For this review, take the finished solid that the model builds, in its own axes (mm). A direction names the side the tool comes from. Give positions to 0.01 mm unless a question says otherwise; leave off trailing zeros. Write each loop counter-clockwise with the first axis right and the second up, starting at its lowest first coordinate (ties: lowest second). Pieces come first, ordered by that corner, then holes.
Q1. We need section D-D (z = 17). Write out the cut boundary in (x, y).
Q2. Insertion check: P1, Ø4, axis at x = 0, z = 24.75, coming from the +Y side; P2, Ø1, axis at y = -1, z = 12.5, coming from the +X side. Each pin has a flat end and moves straight along its axis. Give the tip position at first contact, or say it passes through.
Q3. We need section C-C (z = 24). Write out the cut boundary in (x, y).
Q4. Mouldability with a two-part tool opening along Z and no side actions: class faces 1 (the cylindrical face through (-1.5, 0.02, 0.07)), 2 (the flat face through (0, -1.5, 8)) as released by +Z, released by -Z, zero draft, split by the parting line, or undercut.
Q5. For line 1 (Z direction, x = 0, y = 0.7); line 2 (X direction, y = -0.5, z = -1); line 3 (X direction, y = -0.05, z = 24), list the stretches that pass through material, from the lowest coordinate up.
Q6. We need section A-A (y = 1). Write out the cut boundary in (x, z).
Q7. We need section B-B (x = 0). Write out the cut boundary in (y, z).
Q8. Machinability: for faces 3 (the flat face through (-2.85, -0.02, 11.84)), 4 (the flat face through (2.88, -0.02, 11.52)), 5 (the flat face through (0, 1.5, 8)), which of the approach directions +Z, -Z, +X, -X, +Y, -Y give a long, thin tool a straight path to every point of the face, cutting with its end or side? Answer none if there is none.
```python
from build123d import *

# Parameters (mm, degrees)
F0_R     = 1.5
F1_DEPTH = 1.5


with BuildPart() as f1:
    # F0 (on Front) → F1 (new body, symmetric)
    with BuildSketch(Plane.XZ):
        with BuildLine():
            ThreePointArc((-3.980609, 0.393384), (-0.196931, -3.995149), (4, 0))
            ThreePointArc((4, 0), (3.995149, 0.196931), (3.980609, 0.393384))
            ThreePointArc((3.980609, 0.393384), (0, 4), (-3.980609, 0.393384))
        make_face()
        Circle(F0_R, mode=Mode.SUBTRACT)
        with BuildLine():
            ThreePointArc((-3.980609, 0.393384), (0, 4), (3.980609, 0.393384))
            Line((3.980609, 0.393384), (1.75, 22.964643))
            ThreePointArc((1.75, 22.964643), (0, 22.25), (-1.75, 22.964643))
            Line((-1.75, 22.964643), (-3.980609, 0.393384))
        make_face()
        with BuildLine():
            ThreePointArc((-1.75, 22.964643), (0, 22.25), (1.75, 22.964643))
            ThreePointArc((1.75, 22.964643), (2.304886, 23.781754), (2.5, 24.75))
            ThreePointArc((2.5, 24.75), (-0.968246, 27.054886), (-1.75, 22.964643))
        make_face()
        with Locations((0, 24.75)):
            Circle(F0_R, mode=Mode.SUBTRACT)
    extrude(amount=F1_DEPTH, both=True)


solid = f1.part
```
Computed:
1. outline: (-2.34, -1.5) - (2.34, -1.5) - (2.34, 1.5) - (-2.34, 1.5) - close
2. P1: stops at y = 1.5
2. P2: stops at x = 2.83
3. outline: (-2.38, -1.5) - (-1.3, -1.5) - (-1.3, 1.5) - (-2.38, 1.5) - close; (1.3, -1.5) - (2.38, -1.5) - (2.38, 1.5) - (1.3, 1.5) - close
4. face 1: undercut
4. face 2: zero draft
5. line 1: z = -4 to -1.5, 1.5 to 23.25, 26.25 to 27.25
5. line 2: x = -3.87 to -1.12, 1.12 to 3.87
5. line 3: x = -2.38 to -1.3, 1.3 to 2.38
6. outline: (-3.98, 0.39) arc R4 ccw (long way) to (4, 0) arc R4 ccw to (3.98, 0.39) - (1.75, 22.96) arc R2.5 ccw (long way) to (-1.75, 22.96) - close; hole circle Ø3 at (0, 0); hole circle Ø3 at (0, 24.75)
7. outline: (-1.5, -4) - (1.5, -4) - (1.5, -1.5) - (-1.5, -1.5) - close; (-1.5, 1.5) - (1.5, 1.5) - (1.5, 23.25) - (-1.5, 23.25) - close; (-1.5, 26.25) - (1.5, 26.25) - (1.5, 27.25) - (-1.5, 27.25) - close
8. face 3: -X, +Y, -Y
8. face 4: +X, +Y, -Y
8. face 5: +Z, -Z, +X, -X, +Y
